Verification items for this drawing (mm, ordinates from the low corner). A direction names the side the tool comes from. Coordinates: 2 decimals unless noted, no trailing zeros. Write each loop counter-clockwise with the first axis right and the second up, starting at its lowest first coordinate (ties: lowest second). Pieces come first, ordered by that corner, then holes. Notation, with made-up numbers: M 48.5,67 L 82.5,67 A11 ccw 82.5,76 Z; hole C 20,-26 d6. An arc over 180 degrees is marked long. Answer as CSV lines item,"result". Start each with the question number.
1) Draft check along Y on the marked faces 6, 7, 8 and 9. Enter one of: +Y half, -Y half, draft (parallel to the pull), parting line (faces both ways), or undercut.
2) Access from +Z, -Z, +X, -X, +Y, -Y to the whole of each face (thin tool, end or side, straight path). Record for the marked faces 1, 2, 3, 4 and 5.
3) Section check A-A (z = 3.5). State how many separate pieces and enclosed holes the cut face has, and give its area (3 significant figures).
4) Section check B-B (x = 23.5). Record the cut outline in (y, z).
5) Material ranges on L1, parallel to Y at x = 22, z = 4.25; L2, parallel to Y at x = 39, z = 4.5; L3, parallel to Y at x = 35, z = 0.5 (1 decimal), recorded low to high. Write a range as [from, to].
6) Go/stop test with flat-tipped pins: pin 1 Ø4 at (x, y) = (38, 32.5) entering from -Z; pin 2 Ø5 at (x, y) = (9.5, 21) entering from +Z; pin 3 Ø3 at (y, z) = (9, 4.5) entering from -X. Record where each tip stops, or that it passes through.
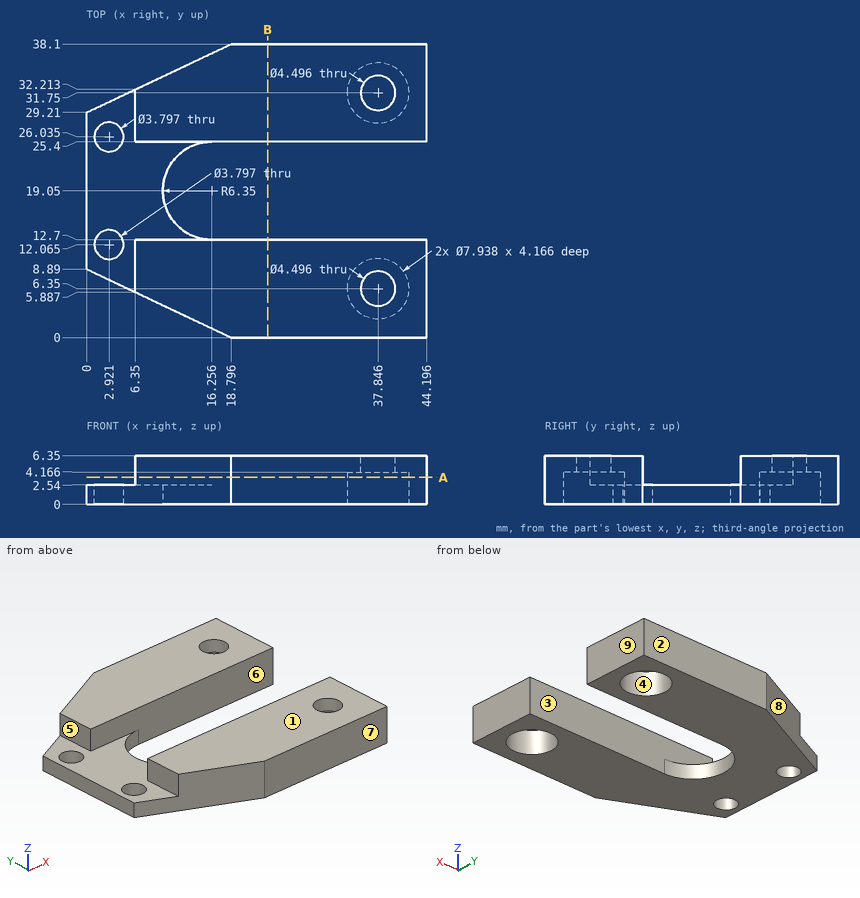
Results found:
1,face 6,"undercut"
1,face 7,"-Y half"
1,face 8,"+Y half"
1,face 9,"draft"
2,face 1,"+Z, +X, -X, +Y, -Y"
2,face 2,"+Z, -Z, +X, -X, +Y"
2,face 3,"+Z, +X"
2,face 4,"-Z"
2,face 5,"+Z, -X, +Y, -Y"
3,separate pieces,"2"
3,enclosed holes,"2"
3,area,"789 mm2"
4,outline,"M 0,0 L 12.7,0 L 12.7,6.35 L 0,6.35 Z; M 25.4,0 L 38.1,0 L 38.1,6.35 L 25.4,6.35 Z"
5,L1,"y = [0, 12.7], [25.4, 38.1]"
5,L2,"y = [0, 4.42], [8.28, 12.7], [25.4, 29.82], [33.68, 38.1]"
5,L3,"y = [0, 3.6], [9.1, 12.7], [25.4, 29], [34.5, 38.1]"
6,pin 1,"stops at z = 4.17"
6,pin 2,"stops at z = 2.54"
6,pin 3,"stops at x = 6.35"
